Drawing for the job (mm, zero at the part's lowest x, y, z). A direction names the side the tool comes from. Round coordinates to 2 decimals unless told otherwise and drop trailing zeros. Write each loop counter-clockwise with the first axis right and the second up, starting at its lowest first coordinate (ties: lowest second). Pieces come first, ordered by that corner, then holes.
Item 1: 3-axis set-ups, long thin cutter, end or side, ignore diameter. For the marked faces 1, 2 and 3: which of +Z, -Z, +X, -X, +Y, -Y reach the whole face in a straight line?
Item 2: Band-saw the part on D-D, the plane z = 9.25. Write the cut outline in (x, y) (1 decimal).
Item 3: Drop flat-ended pins along their axis: pin 1 Ø2 at (x, y) = (19.5, 3.5) entering from -Z (1 decimal); pin 2 Ø3.5 at (x, y) = (94, 19.5) entering from -Z; pin 3 Ø13.5 at (x, y) = (7, 20) entering from -Z (1 decimal); pin 4 Ø3.5 at (x, y) = (10, 22) entering from -Z. Give the stop position or say it passes through.
Item 4: Band-saw the part on C-C, the plane y = 22. Count the separate pieces of the cut face and the enclosed holes in it.
Item 5: Mould opens along X. For the marked faces 4, 5, 6 and 7 say: +X half, -X half, draft (parallel to the pull), parting line (faces both ways), or undercut.
Item 6: Wall check: probe 1 along Y at (x, z) = (10, 24.2); probe 2 along X at (y, z) = (17.5, 13.25) (1 decimal); probe 3 along Z at (x, y) = (88, 4.5). Give the ranges that are in metal, low to high.
Item 7: Band-saw the part on A-A, the plane z = 23.25. Write the cut outline in (x, y) (1 decimal), then the cut area to 3 significant figures.
Item 8: Band-saw the part on B-B, the plane x = 10. Write the cut outline in (y, z), then the cut area to 3 significant figures.
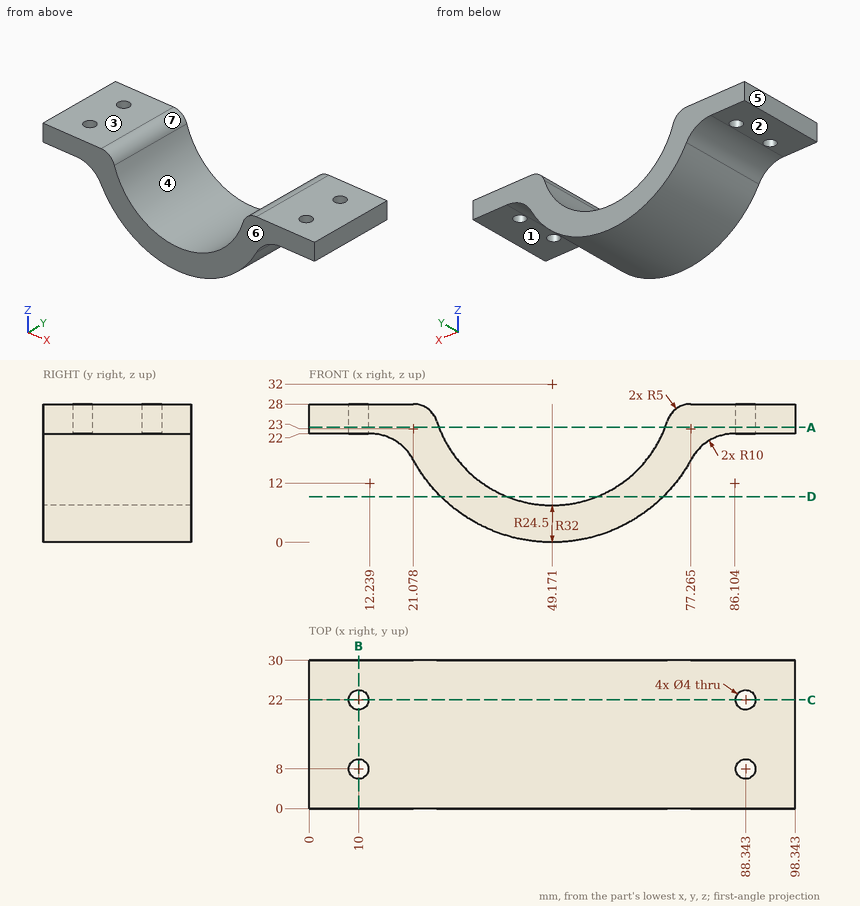
Results:
1. face 1: -Z, +X, +Y, -Y
1. face 2: -Z, -X, +Y, -Y
1. face 3: +Z, +X, -X, +Y, -Y
2. outline: (26.7, 0) - (40.1, 0) - (40.1, 30) - (26.7, 30) - close; (58.3, 0) - (71.7, 0) - (71.7, 30) - (58.3, 30) - close
3. pin 1: stops at z = 17.6
3. pin 2: stops at z = 22
3. pin 3: stops at z = 21.9
3. pin 4: passes through
4. separate pieces: 3
4. enclosed holes: 0
5. face 4: undercut
5. face 5: -X half
5. face 6: draft
5. face 7: undercut
6. probe 1: y = 0 to 6, 10 to 20, 24 to 30
6. probe 2: x = 23.2 to 33.4, 64.9 to 75.1
6. probe 3: z = 22 to 28
7. outline: (0, 0) - (26.3, 0) - (26.3, 30) - (0, 30) - close; (72.1, 0) - (98.3, 0) - (98.3, 30) - (72.1, 30) - close; hole circle Ø4 at (10, 8); hole circle Ø4 at (10, 22); hole circle Ø4 at (88.3, 8); hole circle Ø4 at (88.3, 22)
7. area: 1,530 mm2
8. outline: (0, 22) - (6, 22) - (6, 28) - (0, 28) - close; (10, 22) - (20, 22) - (20, 28) - (10, 28) - close; (24, 22) - (30, 22) - (30, 28) - (24, 28) - close
8. area: 132 mm2
